Work out the finished part from the listing and answer in its coordinate system (mm). A direction names the side the tool comes from. Coordinates: 2 decimals unless noted, no trailing zeros. Order: outer loops, then holes, each group sorted by start corner. A loop starts at its lowest first (then second) coordinate and runs counter-clockwise, first axis right, second up. Notation, with made-up numbers: M -26,33 L -21,33 A26 ccw -21,72 Z; hole C 40,40 d7. An arc over 180 degrees is marked long. Use a Markdown table: item, result.
from build123d import *

# Parameters (mm, degrees)
EXTRUDE_1_DEPTH     = 30.9
CHAMFER_1_SIZE      = 0.5
CUT_EXTRUDE_1_DEPTH = 0.3
SKETCH_6_W          = 0.2
SKETCH_6_H          = 4.8
CUT_EXTRUDE_2_DEPTH = 8.3
CHAMFER_2_SIZE      = 1
CHAMFER_3_SIZE      = 0.6
CHAMFER_4_SIZE      = 0.5
SKETCH_7_R          = 0.4
CUT_EXTRUDE_3_DEPTH = 21.3


with BuildPart() as part:
    # 草图1 → 凸台-拉伸1 (new body)
    with BuildSketch(Plane.XY):
        Polygon((-10, 0), (-10, 7.5), (10, 7.5), (10, 0), (4.5, 0), (4.5, 1), (4.146446609, 1.353553391), (3.646446609, 1.353553391), (3.646446609, 1.853553391), (4.146446609, 1.853553391), (4.5, 2.207106781), (4.5, 4), (-4.5, 4), (-4.5, 2.207106781), (-4.146446609, 1.853553391), (-3.646446609, 1.853553391), (-3.646446609, 1.353553391), (-4.146446609, 1.353553391), (-4.5, 1), (-4.5, 0), align=None)
    extrude(amount=-EXTRUDE_1_DEPTH)

    # 草图3 → M3 螺纹孔1 (revolve, cut)
    with BuildSketch(Plane(origin=(7.5, 7.5, -20.45), x_dir=(0, 0, 1), z_dir=(1, 0, 0))):
        Polygon((0, 0), (0, 3.751075774), (1.25, 3), (1.25, 0), align=None)
    hole_wizard_m3_1 = revolve(axis=Axis((7.5, 13.85, -20.45), (0, -1, 0)), mode=Mode.SUBTRACT)

    # 镜向1: M3 螺纹孔1 across plane
    add(hole_wizard_m3_1.mirror(Plane(origin=(0, 0, -15.45), x_dir=(1, 0, 0), z_dir=(0, 0, -1))), mode=Mode.SUBTRACT)

    # 镜向2: M3 螺纹孔1 across plane
    add(hole_wizard_m3_1.mirror(Plane.ZY), mode=Mode.SUBTRACT)

    # 镜向2 copy 1 sketch → 镜向2 copy 1 (revolve, cut)
    with BuildSketch(Plane(origin=(-7.5, 7.5, -10.45), x_dir=(0, 0, -1), z_dir=(-1, 0, 0))):
        Polygon((0, 0), (0, 3.751075774), (1.25, 3), (1.25, 0), align=None)
    revolve(axis=Axis((-7.5, 13.85, -10.45), (0, -1, 0)), mode=Mode.SUBTRACT)

    # 倒角1
    chamfer_1_edges = [part.edges().sort_by_distance(p)[0] for p in [
        (10, 7.5, -15.45),
        (-10, 7.5, -15.45),
    ]]
    chamfer(chamfer_1_edges, length=CHAMFER_1_SIZE)

    # 草图5 → 切除-拉伸1 (cut)
    with BuildSketch(Plane(origin=(0, 7.5, 0), x_dir=(1, 0, 0), z_dir=(0, 1, 0))):
        Polygon((-9.5, 26.1), (-4.368581018, 26.1), (-4.368581018, 4.8), (-9.5, 4.8), (-10, 4.8), (-10, 0), (10, 0), (10, 4.8), (9.5, 4.8), (4.368581018, 4.8), (4.368581018, 26.1), (9.5, 26.1), (10, 26.1), (10, 30.9), (-10, 30.9), (-10, 26.1), align=None)
    extrude(amount=-CUT_EXTRUDE_1_DEPTH, mode=Mode.SUBTRACT)

    # 草图6 → 切除-拉伸2 (cut)
    with BuildSketch(Plane(origin=(0, 7.2, 0), x_dir=(1, 0, 0), z_dir=(0, 1, 0))):
        with Locations((-9.9, 28.5)):
            Rectangle(SKETCH_6_W, SKETCH_6_H)
        with Locations((9.9, 28.5)):
            Rectangle(SKETCH_6_W, SKETCH_6_H)
        with Locations((9.9, 2.4)):
            Rectangle(SKETCH_6_W, SKETCH_6_H)
        with Locations((-9.9, 2.4)):
            Rectangle(SKETCH_6_W, SKETCH_6_H)
    extrude(amount=-CUT_EXTRUDE_2_DEPTH, mode=Mode.SUBTRACT)

    # 倒角2
    # the kernel refuses this chamfer: 1 mm, written as the material it takes off along each edge
    with BuildSketch(Plane(origin=(-9.8, 7.2, -4.8), x_dir=(-0.027495876610583895, -0.9996219169112968, 0), z_dir=(0, 0, 1)), Plane(origin=(-9.8, 7.2, -33.471682988), x_dir=(-0.027495876610585623, -0.9996219169112968, 0), z_dir=(0, 0, 1))) as chamfer_2_piece_1:
        Polygon((CHAMFER_2_SIZE * 0.999621916911, CHAMFER_2_SIZE * 0.0274958766106), (-CHAMFER_2_SIZE * 0.0274958766106, CHAMFER_2_SIZE * 0.999621916911), (0, 0), align=None)
    extrude(amount=7.371682988, mode=Mode.SUBTRACT)
    with BuildSketch(Plane(origin=(9.8, 7.2, 2.571682988), x_dir=(-0.9996219169112968, 0.02749587661058651, 0), z_dir=(0, 0, -1)), Plane(origin=(9.8, 7.2, -26.1), x_dir=(-0.9996219169112968, 0.02749587661058651, 0), z_dir=(0, 0, -1))) as chamfer_2_piece_2:
        Polygon((CHAMFER_2_SIZE * 0.999621916911, -CHAMFER_2_SIZE * 0.0274958766106), (-CHAMFER_2_SIZE * 0.0274958766106, -CHAMFER_2_SIZE * 0.999621916911), (0, 0), align=None)
    extrude(amount=7.371682988, mode=Mode.SUBTRACT)

    # 倒角3
    chamfer_3_edges = [part.edges().sort_by_distance(p)[0] for p in [
        (-9.8, 0, -28.5),
        (9.8, 0, -28.5),
        (9.8, 0, -2.4),
        (-9.8, 0, -2.4),
    ]]
    chamfer(chamfer_3_edges, length=CHAMFER_3_SIZE)

    # 倒角4
    chamfer_4_edges = [part.edges().sort_by_distance(p)[0] for p in [
        (-10, 0, -15.45),
        (10, 0, -15.45),
    ]]
    chamfer(chamfer_4_edges, length=CHAMFER_4_SIZE)

    # 草图7 → 切除-拉伸3 (cut)
    with BuildSketch(Plane(origin=(0, 0, -26.1), x_dir=(-1, 0, 0), z_dir=(0, 0, -1))):
        with Locations((-10.2, 4)):
            Circle(SKETCH_7_R)
    extrude(amount=-CUT_EXTRUDE_3_DEPTH, mode=Mode.SUBTRACT)


solid = part.part
1. Section C-C on z = -27 is taken. Determine the outline of the cut face in (x, y).
Answers below:
| item | result |
|---|---|
| outline | M -9.8,0.6 L -9.2,0 L -4.5,0 L -4.5,1 L -4.15,1.35 L -3.65,1.35 L -3.65,1.85 L -4.15,1.85 L -4.5,2.21 L -4.5,4 L 4.5,4 L 4.5,2.21 L 4.15,1.85 L 3.65,1.85 L 3.65,1.35 L 4.15,1.35 L 4.5,1 L 4.5,0 L 9.2,0 L 9.8,0.6 L 9.8,6.2 L 8.8,7.2 L -8.8,7.2 L -9.8,6.2 Z |
2. Find the intervals of material crossed by probe 1 along X at (y, z) = (6.4, -20.45); probe 2 along Z at (x, y) = (7.5, 5.9); probe 3 along Z at (x, y) = (-8.25, 5.5), in increasing order.
Answers below:
| item | result |
|---|---|
| probe 1 | -10 to -8.75, -6.25 to 6.25, 8.75 to 10 |
| probe 2 | -30.9 to -21.7, -19.2 to -11.7, -9.2 to 0 |
| probe 3 | -30.9 to -21.45, -19.45 to -11.45, -9.45 to 0 |
3. Section A-A on y = 5.75 is taken. Determine the outline of the cut face in (x, z), then the cut area to 3 significant figures.
Answers below:
| item | result |
|---|---|
| outline | M -10,-26.1 L -9.8,-26.1 L -9.8,-30.9 L 9.8,-30.9 L 9.8,-26.1 L 10,-26.1 L 10,-4.8 L 9.8,-4.8 L 9.8,0 L -9.8,0 L -9.8,-4.8 L -10,-4.8 Z; hole C -7.5,-20.45 d2.5; hole C -7.5,-10.45 d2.5; hole C 7.5,-20.45 d2.5; hole C 7.5,-10.45 d2.5 |
| area | 595 mm² |
4. Flat-ended cylindrical pins translate along their axes: P1, Ø1.4, axis at y = 3.5, z = -27.5, coming from the -X side; P2, Ø1, axis at x = 0.5, z = -21.5, coming from the +Y side. Find the tip coordinate at first contact, or state that the pin passes through.
Answers below:
| item | result |
|---|---|
| P1 | x = -9.8 |
| P2 | y = 7.2 |
5. For faces 1 (the face through (9, 7, -2)), 2 (the face through (-4.5, 0.5, -15.2)), 3 (the face through (4.5, 3, -15)), 4 (the face through (9.8, 3, -2)), 5 (the face through (-9, 7, -2)), determine the directions among +Z, -Z, +X, -X, +Y, -Y from which every point of the face is accessible in a straight line to the end or side of a thin tool.
Answers below:
| item | result |
|---|---|
| face 1 | +Z, +X, +Y |
| face 2 | +Z, -Z, -Y |
| face 3 | +Z, -Z |
| face 4 | +Z, +X, +Y, -Y |
| face 5 | +Z, -X, +Y |
6. For a pull along Z with two mould halves and no side action, classify faces 6 (the face through (7.979, 6.021, -11.605)), 7 (the face through (0.1, 4.5, 0)), 8 (the face through (-7, 7.5, -15)) as +Z half, -Z half, draft (parallel to the pull), parting line (faces both ways), or undercut.
Answers below:
| item | result |
|---|---|
| face 6 | undercut |
| face 7 | +Z half |
| face 8 | draft |
